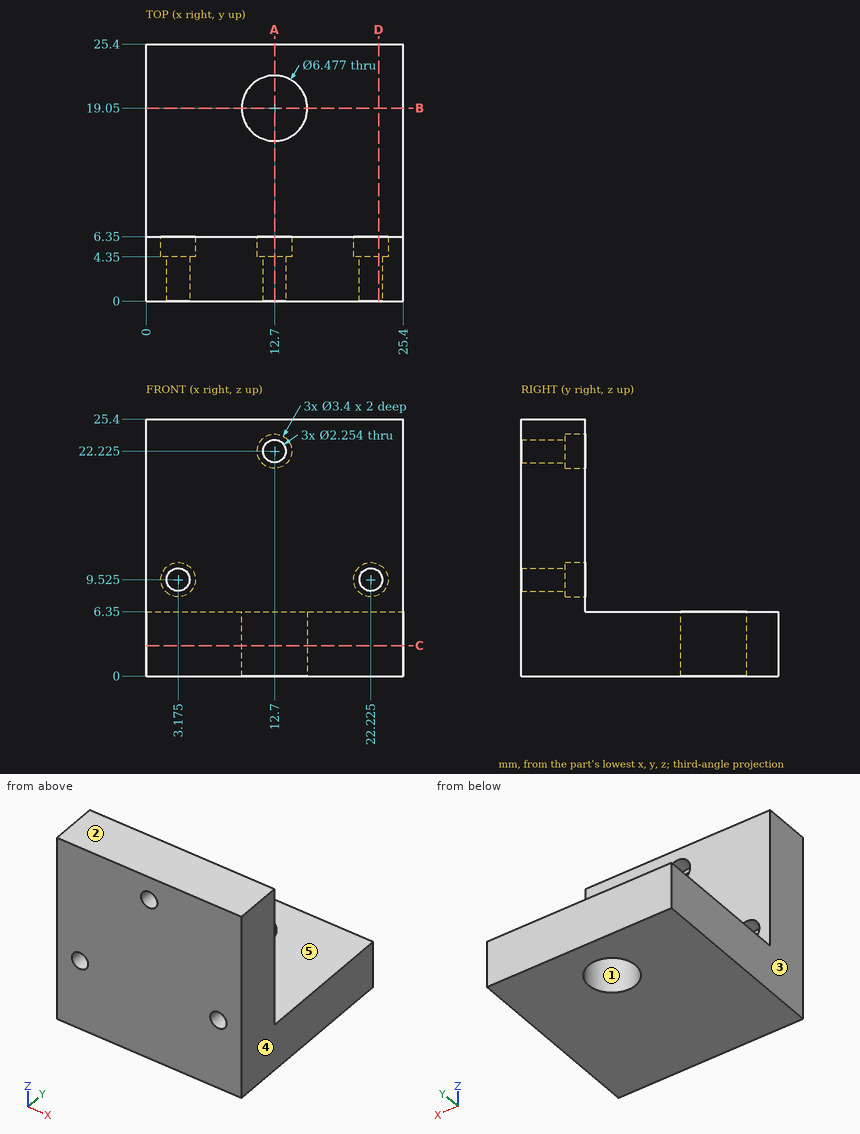
The figure shows three views and two pictorial views of one solid part (mm, origin at its lowest corner). Answer the questions. A direction names the side the tool comes from. Coordinates: 2 decimals unless noted, no trailing zeros. Loops run counter-clockwise (first coordinate to the right, second up) from the corner with the lowest first, then second, coordinate; pieces in that order, holes last.
(1) The part is cut by section B-B (y = 19.05). Determine the outline of the cut face in (x, z), and give its area (3 significant figures).
Solution:
outline: (0, 0) - (9.46, 0) - (9.46, 6.35) - (0, 6.35) - close; (15.94, 0) - (25.4, 0) - (25.4, 6.35) - (15.94, 6.35) - close
area: 120 mm2
(2) The part is cut by section A-A (x = 12.7). Count the separate pieces of the cut face and the enclosed holes in it, and give its area (3 significant figures).
Solution:
separate pieces: 3
enclosed holes: 0
area: 225 mm2
(3) The part is cut by section C-C (z = 3). Determine the outline of the cut face in (x, y).
Solution:
outline: (0, 0) - (25.4, 0) - (25.4, 25.4) - (0, 25.4) - close; hole circle Ø6.48 at (12.7, 19.05)
(4) A tool of negligible diameter and unlimited length cuts with its end or side. For the marked faces 4 and 5, from which of +Z, -Z, +X, -X, +Y, -Y can it reach the whole face along a straight path? Write none if from no direction.
Solution:
face 4: +Z, -Z, +X, +Y, -Y
face 5: +Z, +X, -X, +Y
(5) Consider line 1 along Z through (x, y) = (12.7, 1.8); line 2 along Z through (x, y) = (12.7, 5.55) (3 decimals); line 3 along Y through (x, z) = (15.5, 19.25). Determine where each line is inside the solid, lowest interval first.
Solution:
line 1: z = 0 to 21.1, 23.35 to 25.4
line 2: z = 0 to 20.525, 23.925 to 25.4
line 3: y = 0 to 6.35
(6) Flat-ended cylindrical pins translate along their axes: pin 1 Ø3.5 at (x, z) = (13.5, 22.5) entering from +Y; pin 2 Ø3 at (x, z) = (22.225, 9.525) entering from +Y; pin 3 Ø15 at (x, y) = (10, 17) entering from +Z. Find the tip coordinate at first contact, or state that the pin passes through.
Solution:
pin 1: stops at y = 6.35
pin 2: stops at y = 4.35
pin 3: stops at z = 6.35
(7) The mould has two halves that part along X. Classify the marked faces 1, 2 and 3: released by +X, released by -X, zero draft, split by the parting line, or undercut.
Solution:
face 1: undercut
face 2: zero draft
face 3: released by -X
(8) The part is cut by section D-D (x = 23). Determine the outline of the cut face in (y, z).
Solution:
outline: (0, 0) - (25.4, 0) - (25.4, 6.35) - (6.35, 6.35) - (6.35, 8.01) - (4.35, 8.01) - (4.35, 8.71) - (0, 8.71) - close; (0, 10.34) - (4.35, 10.34) - (4.35, 11.04) - (6.35, 11.04) - (6.35, 25.4) - (0, 25.4) - close
